The listing builds one solid part. Answer for the finished solid, in the listing's coordinates (mm). A direction names the side the tool comes from. Round coordinates to 2 decimals unless told otherwise and drop trailing zeros. Write each loop counter-clockwise with the first axis right and the second up, starting at its lowest first coordinate (ties: lowest second). Pieces come first, ordered by that corner, then holes. Notation, with made-up numbers: (86.25, 82.5) - (99.25, 82.5) arc R22 ccw to (99.25, 110.5) - close; hole circle Ø6 at (-34.75, 82.5). An arc over 180 degrees is marked (long way). Answer as CSV lines item,"result". Start each with the question number.
Item 1: Which of the six approach directions +Z, -Z, +X, -X, +Y, -Y give full straight-line access (tool end or side, diameter ignored) to faces 1 (the cylindrical face through (165.29, 42.73, 22.6)), 2 (the flat face through (56, 10, 18)), 3 (the flat face through (-152, 0, 24))?
Item 2: Straight lines are drawn through the part: line 1 along X through (y, z) = (-22.5, 25.75); line 2 along X through (y, z) = (5.5, 24); line 3 along Y through (x, z) = (-35, 19). For each, find the intervals that lie inside material, in ascending order. Write a range as [from, to].
Item 3: Flat-ended cylindrical pins translate along their axes: pin 1 (9 mm diameter, centred on x = 143.5, y = -8.5, fed in from -Z); pin 2 (3 mm diameter, centred on x = -17.5, y = -2, fed in from -Z). Find the tip coordinate at first contact, or state that the pin passes through.
Item 4: A cutting plane is placed at B-B on x = 68.5. Determine the outline of the cut face in (y, z), and give its area (3 significant figures).
Item 5: For a pull along Y with two mould halves and no side action, classify faces 4 (the flat face through (-2, 30, 30)), 5 (the flat face through (159, 0, 20)), 6 (the cylindrical face through (-165.29, -42.73, 22.6)) as pulls with the +Y half, pulls with the -Y half, needs draft (parallel to the pull), parting line crosses it, or undercut.
Item 6: A cutting plane is placed at A-A on y = 19. Determine the outline of the cut face in (x, z), and give its area (3 significant figures).
Solid Edge part; units mm, degrees
sketch "Sketch1" plane through (0, 0, 0) normal (0, 0, 1) x (1, 0, 0)
  line L0 (-167, -44.5333) -> (167, -44.5333)
  line L1 (167, -44.5333) -> (167, 44.5333)
  line L2 (167, 44.5333) -> (-167, 44.5333)
  line L3 (-167, 44.5333) -> (-167, -44.5333)
extrude "Protrusion1" add sketch "Sketch1" along normal blind 30
sketch "Sketch2" plane through (0, 0, 30) normal (0, 0, 1) x (1, 0, 0)
  line L0 (-152, -25) -> (-91, -25)
  line L1 (-91, -25) -> (-91, 25)
  line L2 (-91, 25) -> (-152, 25)
  line L3 (-152, 25) -> (-152, -25)
extrude "ExtrudedCutout_1" cut sketch "Sketch2" against normal blind 15
fillet "Round_1" radius 3 4 edges at (-152, 25, 22.5) (-91, 25, 22.5) (-152, -25, 22.5) (-91, -25, 22.5)
sketch "Sketch3" plane through (-121.5, 0, 15) normal (0, 0, 1) x (1, 0, 0)
  circle A0 centre (-27.5, 22) radius 2
  circle A1 centre (27.5, 22) radius 2
  circle A2 centre (27.5, -22) radius 2
  circle A3 centre (-27.5, -22) radius 2
extrude "Cutout1" cut sketch "Sketch3" against normal through all
sketch "Sketch4" plane through (0, 0, 0) normal (0, 0, -1) x (-1, 0, 0)
  circle A0 centre (149, 22) radius 4
  circle A1 centre (149, -22) radius 4
  circle A2 centre (94, -22) radius 4
  circle A3 centre (94, 22) radius 4
extrude "ExtrudedCutout_14" cut sketch "Sketch4" against normal blind 5
sketch "Sketch5" plane through (-104.5, 0, 15) normal (0, 0, 1) x (1, 0, 0)
  line L0 (-54.5, 10) -> (263.5, 10)
  line L1 (263.5, 10) -> (263.5, -10)
  line L2 (263.5, -10) -> (-54.5, -10)
  line L3 (-54.5, -10) -> (-54.5, 10)
extrude "ExtrudedCutout_2" cut sketch "Sketch5" against normal blind 6 and the other way blind 6
sketch "Sketch6" plane through (-121.5, -17.5, 15) normal (0, 0, 1) x (-1, 0, 0)
  line L0 (-250.5, 15) -> (-250.5, -50)
  line L1 (-250.5, -50) -> (-280.5, -50)
  line L2 (-280.5, -50) -> (-280.5, 15)
  line L3 (-280.5, 15) -> (-250.5, 15)
extrude "ExtrudedCutout_18" cut sketch "Sketch6" along normal mid plane 20
sketch "Sketch7" plane through (-121.5, -17.5, 15) normal (0, 0, 1) x (-1, 0, 0)
  line L0 (-288.5, -20.5) -> (-280.5, -20.5)
  line L1 (-280.5, -20.5) -> (-280.5, -14.5)
  line L2 (-280.5, -14.5) -> (-288.5, -14.5)
  line L3 (-288.5, -14.5) -> (-288.5, -20.5)
extrude "ExtrudedCutout_19" cut sketch "Sketch7" against normal blind 5
fillet "Round_2" radius 3 6 edges at (-159, 10, 15) (-159, -10, 15) (129, -32.5, 15) (159, -32.5, 15) (159, 32.5, 15) (129, 32.5, 15)
pattern_linear "Pattern1" count 4 spacing 71 along (1, 0, 0) of "ExtrudedCutout_1", "Cutout1", "ExtrudedCutout_14"
fillet "Round1" radius 3 4 edges at (-81, 25, 22.5) (-20, 25, 22.5) (-81, -25, 22.5) (-20, -25, 22.5)
fillet "Round2" radius 3 4 edges at (-10, 25, 22.5) (51, 25, 22.5) (-10, -25, 22.5) (51, -25, 22.5)
fillet "Round3" radius 3 4 edges at (61, 25, 22.5) (122, 25, 22.5) (61, -25, 22.5) (122, -25, 22.5)
sketch "Sketch8" plane through (0, 0, 0) normal (0, 0, -1) x (-1, 0, 0)
  line L0 (-167, 44.5333) -> (167, 44.5333)
  line L1 (167, 44.5333) -> (167, -44.5333)
  line L2 (167, -44.5333) -> (-167, -44.5333)
  line L3 (-167, -44.5333) -> (-167, 44.5333)
extrude "ExtrudedCutout_30" cut sketch "Sketch8" against normal blind 15
fillet "Round_6" radius 6 4 edges at (167, 44.5333, 22.5) (167, -44.5333, 22.5) (-167, -44.5333, 22.5) (-167, 44.5333, 22.5)
Geometry says:
1,face 1,"+Z, -Z, +X, +Y"
1,face 2,"-Z"
1,face 3,"+Z, -Z"
2,line 1,"x = [-167, -151.96], [-91.04, -80.96], [-20.04, -9.96], [50.96, 61.04], [121.96, 167]"
2,line 2,"x = [-167, -152], [-91, -81], [-20, -10], [51, 61], [122, 129], [159, 167]"
2,line 3,"y = [-44.53, -25], [25, 44.53]"
3,pin 1,"stops at z = 25"
3,pin 2,"stops at z = 21"
4,outline,"(-44.53, 15) - (-25, 15) - (-25, 30) - (-44.53, 30) - close; (25, 15) - (44.53, 15) - (44.53, 30) - (25, 30) - close"
4,area,"586 mm^2"
5,face 4,"needs draft"
5,face 5,"undercut"
5,face 6,"pulls with the -Y half"
6,outline,"(-167, 15) - (-152, 15) - (-152, 30) - (-167, 30) - close; (-91, 15) - (-81, 15) - (-81, 30) - (-91, 30) - close; (-20, 15) - (-10, 15) - (-10, 30) - (-20, 30) - close; (51, 15) - (61, 15) - (61, 30) - (51, 30) - close; (122, 15) - (129, 15) - (129, 25) - (159, 25) - (159, 15) - (167, 15) - (167, 30) - (122, 30) - close"
6,area,"1,050 mm^2"
